Could you check a few things on this model? Use its own coordinates, in mm. A direction names the side the tool comes from. Round coordinates to 2 decimals unless told otherwise and drop trailing zeros. Write each loop counter-clockwise with the first axis right and the second up, starting at its lowest first coordinate (ties: lowest second). Pieces come first, ordered by that corner, then holes. Notation, with made-up numbers: (-32.5, 9.25) -> (-19.5, 9.25) arc R11 cw to (-19.5, 14.25) -> close; hole circle Ø9 at (65, -5.75). An arc over 180 degrees is marked (long way). Return JSON: item names as keys, results as strings.
from build123d import *

# Parameters (mm, degrees)
EXTRUDE_1_DEPTH     = 10
EXTRUDE_2_DEPTH     = 64.5
CUT_EXTRUDE_1_REACH = 160.264
SKETCH_4_W          = 45.7
SKETCH_4_H          = 21.3
SKETCH_5_R          = 1.4
SKETCH_5_R_2        = 1.3
EXTRUDE_4_DEPTH     = 3
CUT_EXTRUDE_2_REACH = 160.264
SKETCH_6_W          = 15.410459276
SKETCH_6_H          = 6.940839766
EXTRUDE_7_REACH     = 160.264
CUT_EXTRUDE_3_REACH = 193.728
CUT_EXTRUDE_4_REACH = 193.728
CUT_EXTRUDE_5_REACH = 193.728


with BuildPart() as part:
    # 草圖1 → 填料-伸長1 (new body)
    with BuildSketch(Plane.XY):
        Polygon((85.115442282, 119.023705311), (130.547793458, 40.332564766), (120.155488613, 34.332564766), (120.655488613, 33.466539362), (80.655488613, 33.466539362), (51.851130238, 50.096743424), (12.056130238, 119.023705311), align=None)
        Polygon((51.851130238, 50.096743424), (45.007721115, 46.145699324), (80.655488613, 25.564451164), (80.655488613, 33.466539362), align=None)
    extrude(amount=EXTRUDE_1_DEPTH)

    # 草圖2 → 填料-伸長2 (add)
    with BuildSketch(Plane(origin=(0, 0, 0), x_dir=(-1, 0, 0), z_dir=(0, 0, -1))):
        Polygon((-80.655488613, 33.466539362), (-80.655488613, 25.564451164), (-45.007721115, 46.145699324), (-51.851130238, 50.096743424), (-12.056130238, 119.023705311), (-61.552757034, 119.023705311), (-61.552757034, 57.020497378), (-112.252757034, 57.020497378), (-112.252757034, 72.020497378), (-130.547793458, 40.332564766), (-120.155488613, 34.332564766), (-120.655488613, 33.466539362), align=None)
    extrude(amount=EXTRUDE_2_DEPTH)

    # 草圖4 → 除料-伸長1 (cut, up to next)
    with BuildSketch(Plane(origin=(0, 57.020497378, 0), x_dir=(1, 0, 0), z_dir=(0, 1, 0)), mode=Mode.PRIVATE) as cut_extrude_1_sk1:
        with Locations((86.902757034, 10.65)):
            Rectangle(SKETCH_4_W, SKETCH_4_H)
    cut_extrude_1_tool1 = extrude(cut_extrude_1_sk1.sketch, amount=-CUT_EXTRUDE_1_REACH, mode=Mode.PRIVATE) & part.part
    add(cut_extrude_1_tool1.solids().sort_by_distance((86.902757, 57.020497, -10.65))[0], mode=Mode.SUBTRACT)

    # 草圖5 → 填料-伸長4 (add)
    # profile 1 of 2: a face of its own
    with BuildSketch(Plane(origin=(0, 57.020497378, 0), x_dir=(1, 0, 0), z_dir=(0, 1, 0))):
        with BuildLine():
            Line((64.052757034, 6), (64.052757034, 0))
            Line((64.052757034, 0), (70.052757034, 0))
            Line((70.052757034, 0), (70.052757034, 4.5))
            ThreePointArc((70.052757034, 4.5), (69.613417206, 5.560660172), (68.552757034, 6))
            Line((68.552757034, 6), (64.052757034, 6))
        make_face()
        with Locations(Location((66.552757034, 2.5, 0), (0, 0, 180))):
            Circle(SKETCH_5_R, mode=Mode.SUBTRACT)
    # profile 2 of 2: a face of its own
    with BuildSketch(Plane(origin=(0, 57.020497378, 0), x_dir=(1, 0, 0), z_dir=(0, 1, 0))):
        with BuildLine():
            Line((109.752757034, 15.3), (109.752757034, 21.3))
            Line((109.752757034, 21.3), (103.752757034, 21.3))
            Line((103.752757034, 21.3), (103.752757034, 16.8))
            ThreePointArc((103.752757034, 16.8), (104.192096863, 15.739339828), (105.252757034, 15.3))
            Line((105.252757034, 15.3), (109.752757034, 15.3))
        make_face()
        with Locations(Location((107.252757034, 18.8, 0), (0, 0, 180))):
            Circle(SKETCH_5_R_2, mode=Mode.SUBTRACT)
    extrude(amount=-EXTRUDE_4_DEPTH)

    # 草圖6 → 除料-伸長2 (cut, up to next)
    with BuildSketch(Plane(origin=(0, 57.020497378, 0), x_dir=(1, 0, 0), z_dir=(0, 1, 0)), mode=Mode.PRIVATE) as cut_extrude_2_sk1:
        with Locations((87.057792718, 31.382043144)):
            Rectangle(SKETCH_6_W, SKETCH_6_H)
    cut_extrude_2_tool1 = extrude(cut_extrude_2_sk1.sketch, amount=-CUT_EXTRUDE_2_REACH, mode=Mode.PRIVATE) & part.part
    add(cut_extrude_2_tool1.solids().sort_by_distance((87.057793, 57.020497, -31.382043))[0], mode=Mode.SUBTRACT)

    # 填料-伸長7: up to this face of the body (flat: up to its plane)
    extrude_7_end = Plane(part.part.faces().sort_by_distance((38.998451389, 119.023705311, -25.313032677))[0])
    # 草圖7 → 填料-伸長7 (add, up to the picked face)
    with BuildSketch(Plane(origin=(0, 57.020497378, 0), x_dir=(1, 0, 0), z_dir=(0, 1, 0)), mode=Mode.PRIVATE) as extrude_7_sk1:
        Polygon((94.763022356, 34.85318293), (94.763022356, 22.563502169), (112.252757034, 22.563502169), (112.252757034, 64.5), (61.552757034, 64.5), (61.552757034, 22.563502169), (79.438288953, 22.563502169), (79.35256308, 34.852463027), align=None)
    extrude_7_tool1 = split(extrude(extrude_7_sk1.sketch, amount=EXTRUDE_7_REACH, mode=Mode.PRIVATE), bisect_by=extrude_7_end, keep=Keep.BOTH, mode=Mode.PRIVATE)
    add(extrude_7_tool1.solids().sort_by(Axis((86.885549, 57.020497, -44.976252), (0, 1, 0)))[0])

    # 除料-伸長3: up to this face of the body (flat: up to its plane)
    cut_extrude_3_end = Plane(part.part.faces().sort_by_distance((75.490043398, 78.531685691, -64.5))[0])
    # 草圖9 → 除料-伸長3 (cut, up to the picked face)
    with BuildSketch(Plane.XY.offset(10), mode=Mode.PRIVATE) as cut_extrude_3_sk1:
        Polygon((85.115442282, 119.023705311), (125.857264431, 119.023705311), (125.857264431, 48.688632151), align=None)
    cut_extrude_3_tool1 = split(extrude(cut_extrude_3_sk1.sketch, amount=-CUT_EXTRUDE_3_REACH, mode=Mode.PRIVATE), bisect_by=cut_extrude_3_end, keep=Keep.BOTH, mode=Mode.PRIVATE)
    add(cut_extrude_3_tool1.solids().sort_by(Axis((112.276657, 95.578681, 10), (0, 0, -1)))[0], mode=Mode.SUBTRACT)

    # 草圖10 → 除料-伸長4 (cut, up to next)
    with BuildSketch(Plane(origin=(0, 0, -64.5), x_dir=(-1, 0, 0), z_dir=(0, 0, -1)), mode=Mode.PRIVATE) as cut_extrude_4_sk1:
        Polygon((-120.155488613, 34.332564766), (-118.655488613, 33.466539362), (-120.655488613, 33.466539362), align=None)
    cut_extrude_4_tool1 = extrude(cut_extrude_4_sk1.sketch, amount=-CUT_EXTRUDE_4_REACH, mode=Mode.PRIVATE) & part.part
    add(cut_extrude_4_tool1.solids().sort_by_distance((119.822155, 33.755214, -64.5))[0], mode=Mode.SUBTRACT)

    # 草圖11 → 除料-伸長5 (cut, up to next)
    with BuildSketch(Plane(origin=(0, 0, -64.5), x_dir=(-1, 0, 0), z_dir=(0, 0, -1)), mode=Mode.PRIVATE) as cut_extrude_5_sk1:
        Polygon((-45.007721115, 46.145699324), (-80.655488613, 25.564451164), (-80.655488613, 33.466539362), (-51.851130238, 50.096743424), align=None)
    cut_extrude_5_tool1 = extrude(cut_extrude_5_sk1.sketch, amount=-CUT_EXTRUDE_5_REACH, mode=Mode.PRIVATE) & part.part
    add(cut_extrude_5_tool1.solids().sort_by_distance((64.481905, 38.71348, -64.5))[0], mode=Mode.SUBTRACT)


solid = part.part
1) If I drill on probe 1 along Z at (x, y) = (77, 51); probe 2 along Z at (x, y) = (87.5, 81); probe 3 along X at (y, z) = (55, -2), over which ranges is the centre line in solid material (lowest first)? Write a range as [from, to].
Return value:
{"probe 1": "[-64.5, -21.3], [0, 10]", "probe 2": "[-64.5, -34.85], [0, 10]", "probe 3": "[49.02, 65.25], [67.86, 70.05], [109.75, 122.08]"}
2) Thinking about a two-plate mould opening in Z: for faces 4 (the face through (66.45, 41.67, -27.77)), 5 (the face through (108.55, 55.54, -18.74)), 6 (the face through (72, 77, 10)), which applies, pulls with the +Z half, pulls with the -Z half, needs draft (parallel to the pull), parting line crosses it, or undercut?
Return value:
{"face 4": "needs draft", "face 5": "undercut", "face 6": "pulls with the +Z half"}
3) I want a section at C-C, the plane z = 5.5. Please give me the cut outline in (x, y), and give its area (3 significant figures).
Return value:
{"outline": "(12.06, 119.02) -> (51.85, 50.1) -> (80.66, 33.47) -> (118.66, 33.47) -> (130.55, 40.33) -> (85.12, 119.02) -> close", "area": "6,040 mm²"}
4) Will these pins go through, and if not, where does the flat tip stop? pin 1 Ø6 at (y, z) = (81, -29.5) entering from -X; pin 2 Ø3.5 at (y, z) = (55.5, -3) entering from +X; pin 3 Ø5 at (x, z) = (113, -13) entering from +Y; pin 4 Ø22.5 at (x, z) = (84.5, -9) entering from +Y.
Return value:
{"pin 1": "x = 32.28", "pin 2": "x = 122.8", "pin 3": "y = 72.02", "pin 4": "y = 119.02"}
5) I want a section at A-A, the plane z = -2.5. Please give me the cut outline in (x, y), and give its area (3 significant figures).
Return value:
{"outline": "(12.06, 119.02) -> (51.85, 50.1) -> (64.05, 43.05) -> (64.05, 54.02) -> (65.15, 54.02) -> (65.15, 57.02) -> (61.55, 57.02) -> (61.55, 119.02) -> close; (67.95, 54.02) -> (70.05, 54.02) -> (70.05, 57.02) -> (67.95, 57.02) -> close; (109.75, 33.47) -> (118.66, 33.47) -> (130.55, 40.33) -> (112.25, 72.02) -> (112.25, 57.02) -> (109.75, 57.02) -> close", "area": "2,540 mm²"}
6) I want a section at D-D, the plane x = 83. Count the separate pieces of the cut face and the enclosed holes in it, and give its area (3 significant figures).
Return value:
{"separate pieces": "3", "enclosed holes": "0", "area": "3,550 mm²"}
7) For faces 1 (the face through (70.053, 56, -2)), 2 (the face through (64.053, 50, -11)), 3 (the face through (70, 88, -22.564)), which set-ups out of +Z, -Z, +X, -X, +Y, -Y let a thin tool reach every point of the face, with its end or its side?
Return value:
{"face 1": "+Y, -Y", "face 2": "-Y", "face 3": "+Y"}
8) I want a section at B-B, the plane x = 98. Please give me the cut outline in (y, z).
Return value:
{"outline": "(33.47, -64.5) -> (96.78, -64.5) -> (96.78, -22.56) -> (57.02, -22.56) -> (57.02, -21.3) -> (33.47, -21.3) -> close; (33.47, 0) -> (96.71, 0) -> (96.71, 10) -> (33.47, 10) -> close"}
